Geometry: see drawing. Coordinates: mm, zero at the bounding-box minimum. A direction names the side the tool comes from. Give positions to 0.01 mm unless a question says otherwise; leave off trailing zeros. Write each loop counter-clockwise with the first axis right and the second up, starting at its lowest first coordinate (ties: lowest second). Pieces come first, ordered by that corner, then holes. Notation, with made-up numbers: M 25.5,47.5 L 39.5,47.5 A25 cw 39.5,76.5 Z; hole C 50,-17 d5. An arc over 180 degrees is marked long. Use a Markdown table: item, result. Add a question column.
1) Section B-B on y = 20. Return the cut outline in (x, z), then the cut area to 3 significant figures.
2) Section C-C on z = 4.25. Return the cut outline in (x, y).
3) Line query: line 1 (X direction, y = 25, z = 8); line 2 (Z direction, x = 6, y = 3); line 3 (X direction, y = 3.5, z = 6.75). Output: solid intervals per line, ascending.
4) Section A-A on x = 36. Return the cut outline in (y, z), then the cut area to 3 significant figures.
5) Section D-D on x = 21. Return the cut outline in (y, z).
6) Set-up query: the marked faces 5, 6 and 7. Return all of +Z, -Z, +X, -X, +Y, -Y with unobstructed straight access to the full face (end or side cutting, diameter ignored); none if empty.
7) Draft query along Z for the marked faces 1, 2, 3 and 4. Return one class per face: +Z half, -Z half, draft (parallel to the pull), parting line (faces both ways), or undercut.
8) Pin query (flat end, axial travel): pin 1 (8 mm diameter, centred on y = 15, z = 2, fed in from +X); pin 2 (7 mm diameter, centred on y = 28.5, z = 5, fed in from -X). Return the tip coordinate at first contact, or that it passes through.
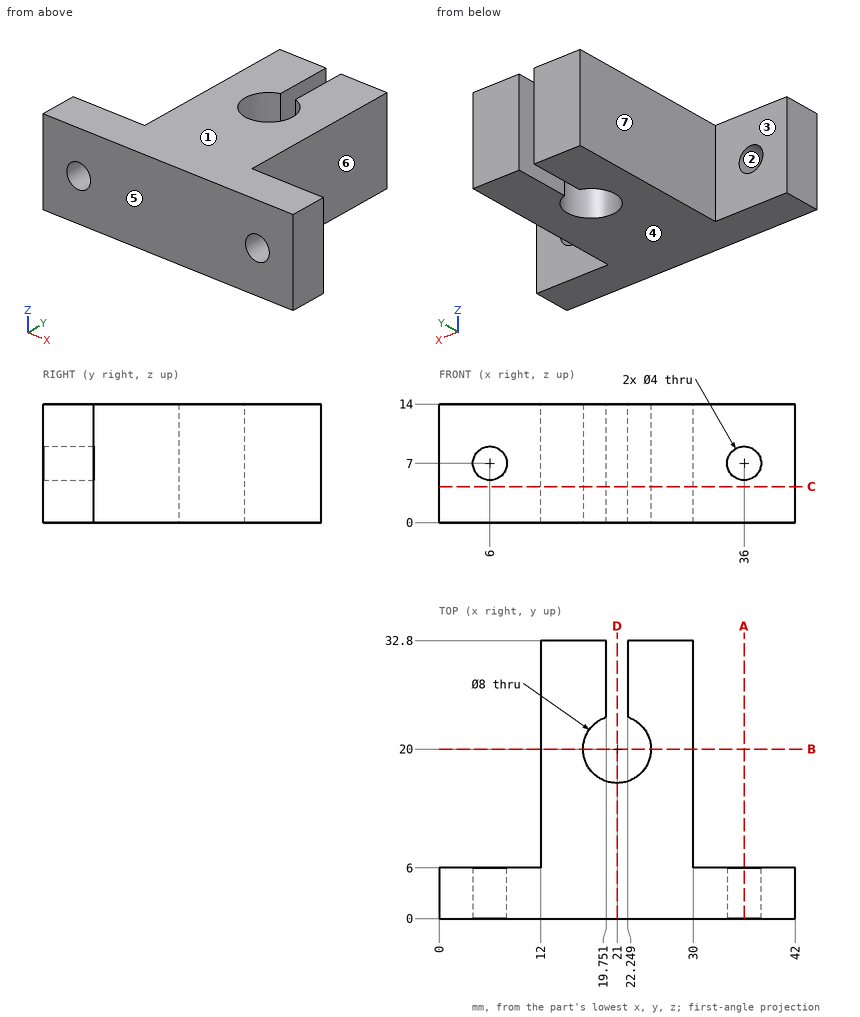
Found:
| question | item | result |
|---|---|---|
| 1 | outline | M 12,0 L 17,0 L 17,14 L 12,14 Z; M 25,0 L 30,0 L 30,14 L 25,14 Z |
| 1 | area | 140 mm² |
| 2 | outline | M 0,0 L 42,0 L 42,6 L 30,6 L 30,32.8 L 22.25,32.8 L 22.25,23.8 A4 cw long 19.75,23.8 L 19.75,32.8 L 12,32.8 L 12,6 L 0,6 Z |
| 3 | line 1 | 12 to 19.75, 22.25 to 30 |
| 3 | line 2 | 0 to 5, 9 to 14 |
| 3 | line 3 | 0 to 4.02, 7.98 to 34.02, 37.98 to 42 |
| 4 | outline | M 0,0 L 6,0 L 6,5 L 0,5 Z; M 0,9 L 6,9 L 6,14 L 0,14 Z |
| 4 | area | 60.0 mm² |
| 5 | outline | M 0,0 L 16,0 L 16,14 L 0,14 Z |
| 6 | face 5 | +Z, -Z, +X, -X, -Y |
| 6 | face 6 | +Z, -Z, +X, +Y |
| 6 | face 7 | +Z, -Z, -X, +Y |
| 7 | face 1 | +Z half |
| 7 | face 2 | undercut |
| 7 | face 3 | draft |
| 7 | face 4 | -Z half |
| 8 | pin 1 | x = 30 |
| 8 | pin 2 | x = 12 |
